```python
from build123d import *

# Parameters (mm, degrees)
SKETCH1_W           = 15
SKETCH1_H           = 35
BOSS_EXTRUDE1_DEPTH = 35
SKETCH3_W           = 8
SKETCH3_H           = 12.2
CUT_EXTRUDE2_DEPTH  = 18
SKETCH4_R           = 1.6
CUT_EXTRUDE3_DEPTH  = 8


with BuildPart() as part:
    # Sketch1 → Boss-Extrude1 (new body)
    with BuildSketch(Plane(origin=(0, 0, 0), x_dir=(1, 0, 0), z_dir=(0, 1, 0))):
        Rectangle(SKETCH1_W, SKETCH1_H)
    extrude(amount=BOSS_EXTRUDE1_DEPTH)

    # Sketch3 → Cut-Extrude2 (cut)
    with BuildSketch(Plane.XY.offset(17.5)):
        with Locations((-3.5, 26.9)):
            Rectangle(SKETCH3_W, SKETCH3_H)
    extrude(amount=-CUT_EXTRUDE2_DEPTH, mode=Mode.SUBTRACT)

    # Sketch4 → Cut-Extrude3 (cut)
    with BuildSketch(Plane(origin=(0, 35, 0), x_dir=(1, 0, 0), z_dir=(0, 1, 0))):
        with Locations(Location((-1.8, -8.5, 0), (0, 0, 270))):  # turned: the seam where the file's is
            Circle(SKETCH4_R)
    extrude(amount=-CUT_EXTRUDE3_DEPTH, mode=Mode.SUBTRACT)


solid = part.part
```
Input: part model. Units: mm. Frame: model coordinates. A direction names the side the tool comes from. Give positions to 0.01 mm unless a question says otherwise; leave off trailing zeros. Order: outer loops, then holes, each group sorted by start corner. A loop starts at its lowest first (then second) coordinate and runs counter-clockwise, first axis right, second up. Notation, with made-up numbers: (58, -16.75) - (70, -16.75) arc R25 cw to (70, -2.75) - close; hole circle Ø10 at (69.25, 19.5). An arc over 180 degrees is marked (long way). One line per item, written item: value.
1. Cut plane A-A, the plane x = -1.8. Output: boundary loops of the cut face in (y, z).
Determined:
outline: (0, -17.5) - (35, -17.5) - (35, 6.9) - (33, 6.9) - (33, -0.5) - (20.8, -0.5) - (20.8, 17.5) - (0, 17.5) - close; (33, 10.1) - (35, 10.1) - (35, 17.5) - (33, 17.5) - close
2. Cut plane B-B, the plane z = 8.5. Output: boundary loops of the cut face in (x, y), and give its area (3 significant figures).
Determined:
outline: (-7.5, 0) - (7.5, 0) - (7.5, 35) - (-0.2, 35) - (-0.2, 33) - (0.5, 33) - (0.5, 20.8) - (-7.5, 20.8) - close; (-7.5, 33) - (-3.4, 33) - (-3.4, 35) - (-7.5, 35) - close
area: 421 mm2
3. Pin query (flat end, axial travel): pin 1 Ø6 at (y, z) = (28.5, 9.5) entering from -X; pin 2 Ø4 at (x, y) = (-2.5, 25.5) entering from +Z. Return the tip coordinate at first contact, or that it passes through.
Determined:
pin 1: x = 0.5
pin 2: z = -0.5
4. Draft query along Z for faces 1 (the face through (0.5, 27, 9)), 2 (the face through (-1.73, 34.01, 6.9)), 3 (the face through (0, 17, -17.5)), 4 (the face through (-4, 27, -0.5)). Return one class per face: released by +Z, released by -Z, zero draft, split by the parting line, or undercut.
Determined:
face 1: zero draft
face 2: undercut
face 3: released by -Z
face 4: released by +Z
5. Cut plane C-C, the plane z = 15.5. Output: boundary loops of the cut face in (x, y), and give its area (3 significant figures).
Determined:
outline: (-7.5, 0) - (7.5, 0) - (7.5, 35) - (-7.5, 35) - (-7.5, 33) - (0.5, 33) - (0.5, 20.8) - (-7.5, 20.8) - close
area: 427 mm2
6. Cut plane D-D, the plane y = 25. Output: boundary loops of the cut face in (x, z).
Determined:
outline: (-7.5, -17.5) - (7.5, -17.5) - (7.5, 17.5) - (0.5, 17.5) - (0.5, -0.5) - (-7.5, -0.5) - close
7. Line query: probe 1 along Y at (x, z) = (-4.25, 16); probe 2 along X at (y, z) = (34.15, 8.5); probe 3 along X at (y, z) = (34, 8). Output: solid intervals per line, ascending.
Determined:
probe 1: 0 to 20.8, 33 to 35
probe 2: -7.5 to -3.4, -0.2 to 7.5
probe 3: -7.5 to -3.32, -0.28 to 7.5
8. Reachability of faces 5 (the face through (2, 13, 17.5)), 6 (the face through (-4, 33, 9)) from +Z, -Z, +X, -X, +Y, -Y: full face, straight path, thin tool, end or side. Return the list, or none.
Determined:
face 5: +Z, +X, -X, +Y, -Y
face 6: +Z, -X
